```python
from build123d import *

# Parameters (mm, degrees)
ESBO_O1_W                = 60
ESBO_O1_H                = 300
RESSALTO_EXTRUS_O1_DEPTH = 3
DOBRA_START              = -30
DOBRA_ESBO_ADA1_DEPTH    = 60
DOBRA_ESBO_ADA1_2_DEPTH  = 60
NERVURA1_START           = -20
NERVURA1_DEPTH           = 40
CORTE_EXTRUS_O1_START    = -175
ESBO_O6_W                = 34
ESBO_O6_H                = 40
CORTE_EXTRUS_O1_DEPTH    = 175
ESBO_O7_R                = 2.5
CORTE_EXTRUS_O2_DEPTH    = 3
ESBO_O8_R                = 6
CORTE_EXTRUS_O3_DEPTH    = 3
ESBO_O9_R                = 2.5
CORTE_EXTRUS_O4_DEPTH    = 3
PADR_OCIRCULAR1_COUNT    = 6


# Read off the part's stored shape, not the designer's step: Dobra esboçada1, Nervura1
with BuildPart() as part:
    # Esboço1 → Ressalto-extrusão1 (new body)
    with BuildSketch(Plane.XY):
        Rectangle(ESBO_O1_W, ESBO_O1_H)
    extrude(amount=RESSALTO_EXTRUS_O1_DEPTH)

    # Dobra esboçada1 outline → Dobra esboçada1 (cut)
    with BuildSketch(Plane.YZ.offset(DOBRA_START)):
        with BuildLine():
            ThreePointArc((99, 3), (101.449489743, 2.16227766), (102.872983346, 0))
            Line((102.872983346, 0), (150, 0))
            Line((150, 0), (150, 3))
            Line((150, 3), (99, 3))
        make_face()
    extrude(amount=DOBRA_ESBO_ADA1_DEPTH, mode=Mode.SUBTRACT)

    # Dobra esbo_ada1 2 outline → Dobra esbo_ada1 2 (add)
    with BuildSketch(Plane.YZ.offset(DOBRA_START)):
        with BuildLine():
            Line((100, -1), (100, -48.073009183))
            Line((100, -48.073009183), (103, -48.073009183))
            Line((103, -48.073009183), (103, -1))
            ThreePointArc((103, -1), (102.968118785, -0.49598283), (102.872983346, 0))
            Line((102.872983346, 0), (99, 0))
            ThreePointArc((99, 0), (99.707106781, -0.292893219), (100, -1))
        make_face()
    extrude(amount=DOBRA_ESBO_ADA1_2_DEPTH)

    # Nervura1 outline → Nervura1 (add)
    with BuildSketch(Plane(origin=(0, 0, 0), x_dir=(0, 0, -1), z_dir=(1, 0, 0)).offset(NERVURA1_START)):
        with BuildLine():
            Line((40, 50), (40, 100))
            Line((40, 100), (1, 100))
            ThreePointArc((1, 100), (0.292893219, 99.707106781), (0, 99))
            Line((0, 99), (0, -75))
            Line((0, -75), (10, -75))
            Line((10, -75), (40, 50))
        make_face()
    extrude(amount=NERVURA1_DEPTH)

    # Esboço6 → Corte-extrusão1 (cut)
    with BuildSketch(Plane.XZ.offset(75).offset(CORTE_EXTRUS_O1_START)):
        with Locations((0, -20)):
            Rectangle(ESBO_O6_W, ESBO_O6_H)
    extrude(amount=CORTE_EXTRUS_O1_DEPTH, mode=Mode.SUBTRACT)

    # Esboço7 → Corte-extrusão2 (cut)
    with BuildSketch(Plane.XY.offset(3)):
        with Locations((-15, -140)):
            Circle(ESBO_O7_R)
        with Locations((15, -140)):
            Circle(ESBO_O7_R)
    extrude(amount=-CORTE_EXTRUS_O2_DEPTH, mode=Mode.SUBTRACT)

    # Esboço8 → Corte-extrusão3 (cut)
    with BuildSketch(Plane(origin=(0, 103, 0), x_dir=(1, 0, 0), z_dir=(0, 1, 0))):
        with Locations(Location((0, 23.073009183, 0), (0, 0, 270))):
            Circle(ESBO_O8_R)
    extrude(amount=-CORTE_EXTRUS_O3_DEPTH, mode=Mode.SUBTRACT)

    # Esboço9 → Corte-extrusão4 (cut)
    with BuildSketch(Plane(origin=(0, 103, 0), x_dir=(1, 0, 0), z_dir=(0, 1, 0))):
        with Locations(Location((0, 35.773009183, 0), (0, 0, 270))):
            Circle(ESBO_O9_R)
    corte_extrus_o4 = extrude(amount=-CORTE_EXTRUS_O4_DEPTH, mode=Mode.SUBTRACT)

    # PadrãoCircular1: Corte-extrusão4 ×6 about axis
    padr_ocircular1_axis = Axis((0, 0, -23.073009183), (0, 1, 0))
    for i in range(1, PADR_OCIRCULAR1_COUNT):
        add(corte_extrus_o4.rotate(padr_ocircular1_axis, i * 360 / PADR_OCIRCULAR1_COUNT), mode=Mode.SUBTRACT)


solid = part.part
```
Design review of the part built by this model. Coordinates are the model's own, in mm. A direction names the side the tool comes from. Coordinates: 2 decimals unless noted, no trailing zeros. Order: outer loops, then holes, each group sorted by start corner. A loop starts at its lowest first (then second) coordinate and runs counter-clockwise, first axis right, second up. Notation, with made-up numbers: (59.25, -31) - (93.25, -31) arc R4 ccw to (93.25, -26) - close; hole circle Ø6 at (-28.75, 63). An arc over 180 degrees is marked (long way). Answer in a Markdown table with one row per item.
(1) Consider section B-B on x = 0. State the section outline as (y, z) points, plus the area to 3 significant figures.
Checked values:
| item | result |
|---|---|
| outline | (-150, 0) - (100, 0) - (100, -7.87) - (103, -7.87) - (103, -1) arc R4 ccw to (99, 3) - (-150, 3) - close; (100, -48.07) - (103, -48.07) - (103, -38.27) - (100, -38.27) - close; (100, -33.27) - (103, -33.27) - (103, -29.07) - (100, -29.07) - close; (100, -17.07) - (103, -17.07) - (103, -12.87) - (100, -12.87) - close |
| area | 834 mm^2 |
(2) Consider section D-D on x = -23.5. State the section outline as (y, z) points, plus the area to 3 significant figures.
Checked values:
| item | result |
|---|---|
| outline | (-150, 0) - (99, 0) arc R1 cw to (100, -1) - (100, -48.07) - (103, -48.07) - (103, -1) arc R4 ccw to (99, 3) - (-150, 3) - close |
| area | 900 mm^2 |
(3) Wall thickness on line 1 along X through (y, z) = (20.5, -32.5); line 2 along Z through (x, y) = (-7.5, -6); line 3 along Y through (x, z) = (-23, -36): over which ranges is each line inside the solid? List them lowest first. Write a range as from..to.
Checked values:
| item | result |
|---|---|
| line 1 | -20..-17, 17..20 |
| line 2 | 0..3 |
| line 3 | 100..103 |
(4) For faces 1 (the flat face through (17, 33, -16)), 2 (the flat face through (20, 33, -15)), 3 (the cylindrical face through (-0.11, 101.521, -7.875)), 4 (the cylindrical face through (14.67, -137.52, 1.52)), 5 (the flat face through (-20, 33, -15)), list the 3-axis set-ups (+Z, -Z, +X, -X, +Y, -Y) from which the entire face can be reached by the end or side of a thin tool; tool diameter is ignored.
Checked values:
| item | result |
|---|---|
| face 1 | -Z, -Y |
| face 2 | -Z, +X, -Y |
| face 3 | +Y, -Y |
| face 4 | +Z, -Z |
| face 5 | -Z, -X, -Y |
(5) Consider section A-A on y = -140. State the section outline as (x, z) points, plus the area to 3 significant figures.
Checked values:
| item | result |
|---|---|
| outline | (-30, 0) - (-17.5, 0) - (-17.5, 3) - (-30, 3) - close; (-12.5, 0) - (12.5, 0) - (12.5, 3) - (-12.5, 3) - close; (17.5, 0) - (30, 0) - (30, 3) - (17.5, 3) - close |
| area | 150 mm^2 |
(6) Clearance check with flat-ended pins moving along their axes: pin 1 (2 mm diameter, centred on x = -15.5, y = -79.5, fed in from -Z); pin 2 (6 mm diameter, centred on x = 0, z = -35.77, fed in from -Y); pin 3 (12 mm diameter, centred on y = 14.5, z = -25.5, fed in from +X); pin 4 (4 mm diameter, centred on x = -15, y = -140, fed in from -Z). State where each tip first meets the part, or that it passes through.
Checked values:
| item | result |
|---|---|
| pin 1 | z = 0 |
| pin 2 | y = 100 |
| pin 3 | x = 20 |
| pin 4 | through |
(7) Consider section C-C on y = -53. State the section outline as (x, z) points.
Checked values:
| item | result |
|---|---|
| outline | (-30, 0) - (-20, 0) - (-20, -15.28) - (-17, -15.28) - (-17, 0) - (17, 0) - (17, -15.28) - (20, -15.28) - (20, 0) - (30, 0) - (30, 3) - (-30, 3) - close |
(8) The part is to be moulded in two halves that separate along Z. For faces 6 (the cylindrical face through (-0.958, 101.521, -33.464)), 7 (the cylindrical face through (-15.33, -137.52, 1.52)), 8 (the flat face through (0, -24, 3)), 9 (the cylindrical face through (-12.52, 101.521, -18.707)), say which applies: released by +Z, released by -Z, zero draft, split by the parting line, or undercut.
Checked values:
| item | result |
|---|---|
| face 6 | undercut |
| face 7 | zero draft |
| face 8 | released by +Z |
| face 9 | undercut |
